Here's how the part is built. I have some questions about the finished solid (model axes, mm). A direction names the side the tool comes from. Round coordinates to 2 decimals unless told otherwise and drop trailing zeros. Loops run counter-clockwise (first coordinate to the right, second up) from the corner with the lowest first, then second, coordinate; pieces in that order, holes last. Notation, with made-up numbers: M -38.5,15.5 L -33.5,15.5 A27 ccw -33.5,51.5 Z; hole C 24.25,75 d6. An arc over 180 degrees is marked long. One line per question, with ' | ' between items. Start each with the question number.
```python
from build123d import *

# Parameters (mm, degrees)
SKETCH1_W                 = 75
SKETCH1_H                 = 40
SKETCH1_R                 = 5
SKETCH1_R_2               = 1.7
SKETCH1_W_2               = 10
SKETCH1_H_2               = 20
BOSS_EXTRUDE1_DEPTH       = 3
CUT_EXTRUDE1_DEPTH        = 43.605750786
CUT_EXTRUDE1_DEPTH_BACK   = 43.605750786
SKETCH2_W                 = 67
SKETCH2_H                 = 28
BOSS_EXTRUDE3_DEPTH       = 110
BOSS_EXTRUDE3_DEPTH_BACK  = 3
SKETCH6_W                 = 67
SKETCH6_H                 = 11
CUT_EXTRUDE4_DEPTH        = 122.372360939
SKETCH7_W                 = 70
SKETCH7_H                 = 37
BOSS_EXTRUDE4_DEPTH       = 45
SKETCH8_W                 = 45
SKETCH8_H                 = 62
CUT_EXTRUDE6_DEPTH        = 29
SKETCH11_W                = 45
SKETCH11_H                = 4
CUT_EXTRUDE9_DEPTH        = 157.445677473
SKETCH9_W                 = 38
SKETCH9_H                 = 28.5
CUT_EXTRUDE10_DEPTH       = 204.024629048
SKETCH13_W                = 5
SKETCH13_H                = 38
BOSS_EXTRUDE5_DEPTH       = 32
SKETCH14_R                = 5
SKETCH14_R_2              = 1.7
CUT_EXTRUDE11_DEPTH       = 32
SKETCH15_W                = 165
SKETCH15_H                = 70
SKETCH15_W_2              = 157
SKETCH15_H_2              = 62
BOSS_EXTRUDE6_DEPTH       = 3
SKETCH16_W                = 20
SKETCH16_H                = 4.820648258
CUT_EXTRUDE12_DEPTH       = 159.626132778
SKETCH18_R                = 5
CUT_EXTRUDE14_DEPTH       = 159.626132778
MIRROR6_COPY_1_SKETCH_W   = 5
MIRROR6_COPY_1_SKETCH_H   = 38
MIRROR6_COPY_1_DEPTH      = 32
MIRROR6_COPY_2_SKETCH_R   = 5
MIRROR6_COPY_2_SKETCH_R_2 = 1.7
MIRROR6_COPY_2_DEPTH      = 32
SKETCH19_W                = 38
SKETCH19_H                = 3.5
CUT_EXTRUDE15_DEPTH       = 10
SKETCH20_R                = 1.2
CUT_EXTRUDE16_DEPTH       = 10
SKETCH21_W                = 10
SKETCH21_H                = 80
CUT_EXTRUDE17_DEPTH       = 184.330984833
SKETCH22_W                = 55
SKETCH22_H                = 80
CUT_EXTRUDE18_DEPTH       = 184.330984833
SKETCH23_W                = 67
SKETCH23_H                = 62
BOSS_EXTRUDE7_DEPTH       = 3
SKETCH24_R                = 10
SKETCH24_R_2              = 2.75
CUT_EXTRUDE19_DEPTH       = 111.707949127
SKETCH25_W                = 38
SKETCH25_H                = 64
CUT_EXTRUDE20_DEPTH       = 115


with BuildPart() as part:
    # Sketch1 → Boss-Extrude1 (new body)
    with BuildSketch(Plane(origin=(0, 0, 0), x_dir=(1, 0, 0), z_dir=(0, 1, 0))):
        Rectangle(SKETCH1_W, SKETCH1_H)
        with Locations(Location((-21, 0, 0), (0, 0, 270))):
            Circle(SKETCH1_R, mode=Mode.SUBTRACT)
        with Locations(Location((-30, 8.25, 0), (0, 0, 270))):
            Circle(SKETCH1_R_2, mode=Mode.SUBTRACT)
        with Locations(Location((-12, 8.25, 0), (0, 0, 270))):
            Circle(SKETCH1_R_2, mode=Mode.SUBTRACT)
        with Locations(Location((-12, -8.25, 0), (0, 0, 270))):
            Circle(SKETCH1_R_2, mode=Mode.SUBTRACT)
        with Locations(Location((-30, -8.25, 0), (0, 0, 270))):
            Circle(SKETCH1_R_2, mode=Mode.SUBTRACT)
        with Locations(Location((12, 8.25, 0), (0, 0, 90))):
            Circle(SKETCH1_R_2, mode=Mode.SUBTRACT)
        with Locations(Location((12, -8.25, 0), (0, 0, 90))):
            Circle(SKETCH1_R_2, mode=Mode.SUBTRACT)
        with Locations(Location((21, 0, 0), (0, 0, 90))):
            Circle(SKETCH1_R, mode=Mode.SUBTRACT)
        with Locations(Location((30, -8.25, 0), (0, 0, 90))):
            Circle(SKETCH1_R_2, mode=Mode.SUBTRACT)
        with Locations(Location((30, 8.25, 0), (0, 0, 90))):
            Circle(SKETCH1_R_2, mode=Mode.SUBTRACT)
        Rectangle(SKETCH1_W_2, SKETCH1_H_2, mode=Mode.SUBTRACT)
    extrude(amount=BOSS_EXTRUDE1_DEPTH)

    # Sketch2 → Cut-Extrude1 (cut, two sides: drawn at the far end of the back side and taken through both)
    with BuildSketch(Plane(origin=(0, 3, 0), x_dir=(1, 0, 0), z_dir=(0, 1, 0)).offset(-CUT_EXTRUDE1_DEPTH_BACK)):
        Rectangle(SKETCH2_W, SKETCH2_H)
    extrude(amount=CUT_EXTRUDE1_DEPTH + CUT_EXTRUDE1_DEPTH_BACK, mode=Mode.SUBTRACT)

    # Sketch3 → Boss-Extrude3 (add, two sides: drawn at the far end of the back side and taken through both)
    with BuildSketch(Plane(origin=(0, 3, 0), x_dir=(1, 0, 0), z_dir=(0, 1, 0)).offset(-BOSS_EXTRUDE3_DEPTH_BACK)):
        Polygon((37.5, -35), (37.5, -20), (33.5, -20), (-33.5, -20), (-37.5, -20), (-37.5, -35), align=None)
        Polygon((33.5, 20), (37.5, 20), (37.5, 35), (-37.5, 35), (-37.5, 20), (-33.5, 20), align=None)
        Polygon((37.5, -20), (37.5, 20), (33.5, 20), (33.5, 14), (33.5, -14), (33.5, -20), align=None)
        Polygon((-33.5, 14), (-33.5, 20), (-37.5, 20), (-37.5, -20), (-33.5, -20), (-33.5, -14), align=None)
    extrude(amount=BOSS_EXTRUDE3_DEPTH + BOSS_EXTRUDE3_DEPTH_BACK)

    # Sketch6 → Cut-Extrude4 (cut, through all)
    with BuildSketch(Plane(origin=(0, 3, 0), x_dir=(1, 0, 0), z_dir=(0, 1, 0))):
        with Locations((0, -25.5)):
            Rectangle(SKETCH6_W, SKETCH6_H)
        with Locations((0, 25.5)):
            Rectangle(SKETCH6_W, SKETCH6_H)
    extrude(amount=CUT_EXTRUDE4_DEPTH, mode=Mode.SUBTRACT)

    # Sketch7 → Boss-Extrude4 (add)
    with BuildSketch(Plane.ZY.offset(37.5)):
        with Locations((0, 94.5)):
            Rectangle(SKETCH7_W, SKETCH7_H)
    boss_extrude4 = extrude(amount=BOSS_EXTRUDE4_DEPTH)

    # Mirror2: Boss-Extrude4 across plane
    add(boss_extrude4.mirror(Plane(origin=(0, 0, 0), x_dir=(0, 0, 1), z_dir=(1, 0, 0))))

    # Sketch8 → Cut-Extrude6 (cut)
    with BuildSketch(Plane(origin=(0, 113, 0), x_dir=(1, 0, 0), z_dir=(0, 1, 0))):
        with Locations((-56, 0)):
            Rectangle(SKETCH8_W, SKETCH8_H)
        with Locations((56, 0)):
            Rectangle(SKETCH8_W, SKETCH8_H)
    extrude(amount=-CUT_EXTRUDE6_DEPTH, mode=Mode.SUBTRACT)

    # Sketch11 → Cut-Extrude9 (cut, through all)
    with BuildSketch(Plane.XY.offset(35)):
        with Locations((-60, 78)):
            Rectangle(SKETCH11_W, SKETCH11_H)
        with Locations((60, 78)):
            Rectangle(SKETCH11_W, SKETCH11_H)
    extrude(amount=-CUT_EXTRUDE9_DEPTH, mode=Mode.SUBTRACT)

    # Sketch9 → Cut-Extrude10 (cut, through all)
    with BuildSketch(Plane.ZY.offset(82.5)):
        with Locations((0, 98.25)):
            Rectangle(SKETCH9_W, SKETCH9_H)
    extrude(amount=-CUT_EXTRUDE10_DEPTH, mode=Mode.SUBTRACT)

    # Sketch13 → Boss-Extrude5 (add)
    with BuildSketch(Plane(origin=(0, 84, 0), x_dir=(1, 0, 0), z_dir=(0, 1, 0))):
        with Locations((-54.5, 0)):
            Rectangle(SKETCH13_W, SKETCH13_H)
    boss_extrude5 = extrude(amount=BOSS_EXTRUDE5_DEPTH)

    # Sketch14 → Cut-Extrude11 (cut)
    with BuildSketch(Plane.ZY.offset(57)):
        with Locations((0, 98.25)):
            Circle(SKETCH14_R)
        with Locations((-9, 106.5)):
            Circle(SKETCH14_R_2)
        with Locations((9, 106.5)):
            Circle(SKETCH14_R_2)
        with Locations((9, 90)):
            Circle(SKETCH14_R_2)
        with Locations((-9, 90)):
            Circle(SKETCH14_R_2)
    cut_extrude11 = extrude(amount=-CUT_EXTRUDE11_DEPTH, mode=Mode.SUBTRACT)

    # Mirror4: Boss-Extrude5, Cut-Extrude11 across plane
    add(boss_extrude5.mirror(Plane(origin=(0, 0, 0), x_dir=(0, 0, 1), z_dir=(1, 0, 0))))
    add(cut_extrude11.mirror(Plane(origin=(0, 0, 0), x_dir=(0, 0, 1), z_dir=(1, 0, 0))), mode=Mode.SUBTRACT)

    # Sketch15 → Boss-Extrude6 (add)
    with BuildSketch(Plane(origin=(0, 113, 0), x_dir=(1, 0, 0), z_dir=(0, 1, 0))):
        Rectangle(SKETCH15_W, SKETCH15_H)
        Rectangle(SKETCH15_W_2, SKETCH15_H_2, mode=Mode.SUBTRACT)
    extrude(amount=BOSS_EXTRUDE6_DEPTH)

    # Sketch16 → Cut-Extrude12 (cut, through all)
    with BuildSketch(Plane.XY.offset(35)):
        with Locations((0, 11.636111214)):
            Rectangle(SKETCH16_W, SKETCH16_H)
    extrude(amount=-CUT_EXTRUDE12_DEPTH, mode=Mode.SUBTRACT)

    # Sketch18 → Cut-Extrude14 (cut, through all)
    with BuildSketch(Plane.XY.offset(35)):
        with Locations((67.75, 100)):
            Circle(SKETCH18_R)
    cut_extrude14 = extrude(amount=-CUT_EXTRUDE14_DEPTH, mode=Mode.SUBTRACT)

    # Mirror5: Cut-Extrude14 across plane
    add(cut_extrude14.mirror(Plane(origin=(0, 0, 0), x_dir=(0, 0, 1), z_dir=(1, 0, 0))), mode=Mode.SUBTRACT)

    # Mirror6: Boss-Extrude5, Cut-Extrude11 across plane
    add(boss_extrude5.mirror(Plane.ZX.offset(116)))
    add(cut_extrude11.mirror(Plane.ZX.offset(116)), mode=Mode.SUBTRACT)

    # Mirror6 copy 1 sketch → Mirror6 copy 1 (add)
    with BuildSketch(Plane(origin=(0, 148, 0), x_dir=(-1, 0, 0), z_dir=(0, -1, 0))):
        with Locations((-54.5, 0)):
            Rectangle(MIRROR6_COPY_1_SKETCH_W, MIRROR6_COPY_1_SKETCH_H)
    extrude(amount=MIRROR6_COPY_1_DEPTH)

    # Mirror6 copy 2 sketch → Mirror6 copy 2 (cut)
    with BuildSketch(Plane(origin=(57, 232, 0), x_dir=(0, 0, 1), z_dir=(1, 0, 0))):
        with Locations((0, 98.25)):
            Circle(MIRROR6_COPY_2_SKETCH_R)
        with Locations((-9, 106.5)):
            Circle(MIRROR6_COPY_2_SKETCH_R_2)
        with Locations((9, 106.5)):
            Circle(MIRROR6_COPY_2_SKETCH_R_2)
        with Locations((9, 90)):
            Circle(MIRROR6_COPY_2_SKETCH_R_2)
        with Locations((-9, 90)):
            Circle(MIRROR6_COPY_2_SKETCH_R_2)
    extrude(amount=-MIRROR6_COPY_2_DEPTH, mode=Mode.SUBTRACT)

    # Sketch19 → Cut-Extrude15 (cut)
    with BuildSketch(Plane(origin=(82.5, 0, 0), x_dir=(0, 0, -1), z_dir=(1, 0, 0))):
        with Locations((0, 114.25)):
            Rectangle(SKETCH19_W, SKETCH19_H)
    cut_extrude15 = extrude(amount=-CUT_EXTRUDE15_DEPTH, mode=Mode.SUBTRACT)

    # Mirror7: Cut-Extrude15 across plane
    add(cut_extrude15.mirror(Plane(origin=(0, 0, 0), x_dir=(0, 0, 1), z_dir=(1, 0, 0))), mode=Mode.SUBTRACT)

    # Sketch20 → Cut-Extrude16 (cut)
    with BuildSketch(Plane(origin=(0, 3, 0), x_dir=(1, 0, 0), z_dir=(0, 1, 0))):
        with Locations(Location((-24, 17.5, 0), (0, 0, 270))):
            Circle(SKETCH20_R)
        with Locations(Location((-12, 17.5, 0), (0, 0, 270))):
            Circle(SKETCH20_R)
        with Locations(Location((12, 17.5, 0), (0, 0, 270))):
            Circle(SKETCH20_R)
        with Locations(Location((-24, -17.5, 0), (0, 0, 270))):
            Circle(SKETCH20_R)
        with Locations(Location((-12, -17.5, 0), (0, 0, 270))):
            Circle(SKETCH20_R)
        with Locations(Location((24, 17.5, 0), (0, 0, 270))):
            Circle(SKETCH20_R)
        with Locations(Location((12, -17.5, 0), (0, 0, 270))):
            Circle(SKETCH20_R)
        with Locations(Location((24, -17.5, 0), (0, 0, 270))):
            Circle(SKETCH20_R)
    extrude(amount=-CUT_EXTRUDE16_DEPTH, mode=Mode.SUBTRACT)

    # Sketch21 → Cut-Extrude17 (cut, through all)
    with BuildSketch(Plane.XY.offset(35)):
        with Locations((32.5, 40)):
            Rectangle(SKETCH21_W, SKETCH21_H)
        with Locations((-32.5, 40)):
            Rectangle(SKETCH21_W, SKETCH21_H)
    extrude(amount=-CUT_EXTRUDE17_DEPTH, mode=Mode.SUBTRACT)

    # Sketch22 → Cut-Extrude18 (cut, through all)
    with BuildSketch(Plane.XY.offset(35)):
        with Locations((0, 40)):
            Rectangle(SKETCH22_W, SKETCH22_H)
    extrude(amount=-CUT_EXTRUDE18_DEPTH, mode=Mode.SUBTRACT)

    # Sketch23 → Boss-Extrude7 (add)
    with BuildSketch(Plane.XZ.offset(-80)):
        Rectangle(SKETCH23_W, SKETCH23_H)
    extrude(amount=-BOSS_EXTRUDE7_DEPTH)

    # Sketch24 → Cut-Extrude19 (cut, through all)
    with BuildSketch(Plane(origin=(0, 83, 0), x_dir=(1, 0, 0), z_dir=(0, 1, 0))):
        with Locations(Location((0, 0, 0), (0, 0, 270))):
            Circle(SKETCH24_R)
        with Locations(Location((-20, 19, 0), (0, 0, 270))):
            Circle(SKETCH24_R_2)
        with Locations(Location((-20, -19, 0), (0, 0, 270))):
            Circle(SKETCH24_R_2)
        with Locations(Location((20, -19, 0), (0, 0, 90))):
            Circle(SKETCH24_R_2)
        with Locations(Location((20, 19, 0), (0, 0, 90))):
            Circle(SKETCH24_R_2)
    extrude(amount=-CUT_EXTRUDE19_DEPTH, mode=Mode.SUBTRACT)

    # Sketch25 → Cut-Extrude20 (cut)
    with BuildSketch(Plane(origin=(57, 0, 0), x_dir=(0, 0, -1), z_dir=(1, 0, 0))):
        with Locations((0, 116)):
            Rectangle(SKETCH25_W, SKETCH25_H)
    extrude(amount=-CUT_EXTRUDE20_DEPTH, mode=Mode.SUBTRACT)


solid = part.part
```
1) I'm going to push flat-ended pins straight in: pin 1 Ø4.5 at (x, z) = (-20, -19) entering from -Y; pin 2 Ø24.5 at (x, z) = (-65.5, -3.5) entering from +Y; pin 3 Ø9 at (x, z) = (20, 19) entering from +Y. Where does each tip first touch, or does it pass through?
2) Please list where these lines run through material, in increasing order: L1, parallel to X at y = 81, z = -19; L2, parallel to Z at x = 20, y = 82; L3, parallel to X at y = 90, z = 27.5. Write a range as from..to.
3) Imagine slicing it at B-B (z = 0). Write out the boundary of the cut face in (x, y).
4) For faces 1 (the face through (-19.879, 81.521, -21.747)), 2 (the face through (-1, 99, -31)), which set-ups out of +Z, -Z, +X, -X, +Y, -Y let a thin tool reach every point of the face, with its end or its side?
5) Imagine slicing it at A-A (x = 67.75). Write out the boundary of the cut face in (y, z).
6) Imagine slicing it at C-C (x = -28). Write out the boundary of the cut face in (y, z), then the cut area to 3 significant figures.
7) Imagine slicing it at D-D (z = 13). Write out the boundary of the cut face in (x, y).
8) We'd pull the mould along Y, two halves only. Please class faces 3 (the face through (66.67, 95.12, -32.97)), 4 (the face through (-78.5, 100, -25)), 5 (the face through (0, 116, -32)): pulls with the +Y half, pulls with the -Y half, needs draft (parallel to the pull), parting line crosses it, or undercut.
Results are:
1) pin 1: through | pin 2: y = 84 | pin 3: y = 83
2) L1: -82.5..-22.75, -17.25..17.25, 22.75..82.5 | L2: -35..-21.75, -16.25..16.25, 21.75..35 | L3: -82.5..-78.5, 78.5..82.5
3) outline: M -82.5,80 L -10,80 L -10,83 L -33.5,83 L -33.5,84 L -82.5,84 Z; M 10,80 L 82.5,80 L 82.5,84 L 33.5,84 L 33.5,83 L 10,83 Z
4) face 1: +Y, -Y | face 2: +Y
5) outline: M 80,-35 L 95,-35 L 95,-31 L 84,-31 L 84,31 L 95,31 L 95,35 L 80,35 Z; M 105,-35 L 116,-35 L 116,-31 L 105,-31 Z; M 105,31 L 116,31 L 116,35 L 105,35 Z
6) outline: M 80,-35 L 116,-35 L 116,-31 L 83,-31 L 83,31 L 116,31 L 116,35 L 80,35 Z | area: 474 mm²
7) outline: M -82.5,80 L 82.5,80 L 82.5,84 L 33.5,84 L 33.5,83 L -33.5,83 L -33.5,84 L -82.5,84 Z
8) face 3: undercut | face 4: needs draft | face 5: pulls with the +Y half
